Verification items for the finished model (mm, model axes). Face numbers are marked on the shaded views. Round coordinates to 2 decimals unless told otherwise and drop trailing zeros. Write each loop counter-clockwise with the first axis right and the second up, starting at its lowest first coordinate (ties: lowest second). Pieces come first, ordered by that corner, then holes. Notation, with made-up numbers: (62.25, -9.5) - (75.25, -9.5) arc R24 ccw to (75.25, 21.5) - close; hole circle Ø7 at (64, 19.5). An arc over 180 degrees is marked (long way). Answer as a JSON object with one key per item and string values. Group by question number.
1) Thickness scan on line 1 (X direction, y = -7, z = 2.2) (3 decimals); line 2 (X direction, y = 12.5, z = 2.4); line 3 (X direction, y = -5, z = 0.6). Record the ranges inside material, lowest first.
2) Mould release check, pull along Y, two halves, no side actions. Record for the marked faces 1, 2 and 3: +Y half, -Y half, draft (parallel to the pull), parting line (faces both ways), or undercut.
3) Section check A-A (y = 14). Enter the section's corners in (x, z), then the cut area to 3 significant figures.
4) Go/stop test with a flat-tipped pin: pin 1 Ø6 at (x, y) = (-12.12, -7) entering from +Z. Record where the tip stops, or that it passes through.
5) Section check D-D (x = 0). Enter the section's corners in (y, z), then the cut area to 4 significant figures.
6) Section check C-C (z = 1). Enter the section's corners in (x, y) (3 decimals), then the cut area to 3 significant figures.
7) Section check B-B (x = -11.5). Enter the section's corners in (y, z), then the cut area to 3 significant figures.
```python
from build123d import *

# Parameters (mm, degrees)
BOSS_EXTRU_2_DEPTH = 3


with BuildPart() as part:
    # Esquisse1 → Boss.-Extru.2 (new body)
    with BuildSketch(Plane.XY):
        with BuildLine():
            ThreePointArc((-12.288149304, -10.247018429), (0.000780623, -15.999999981), (12.289149128, -10.245819328))
            ThreePointArc((12.289149128, -10.245819328), (9.309773091, -5.375), (15.017714385, -5.519805672))
            ThreePointArc((15.017714385, -5.519805672), (13.856406461, 8), (2.728565257, 15.765625))
            ThreePointArc((2.728565257, 15.765625), (0, 10.75), (-2.728565257, 15.765625))
            ThreePointArc((-2.728565257, 15.765625), (-13.856384318, 8.000038352), (-15.01774494, -5.519722539))
            ThreePointArc((-15.01774494, -5.519722539), (-9.310492225, -5.375986513), (-12.288149304, -10.247018429))
        make_face()
    extrude(amount=BOSS_EXTRU_2_DEPTH)


solid = part.part
```
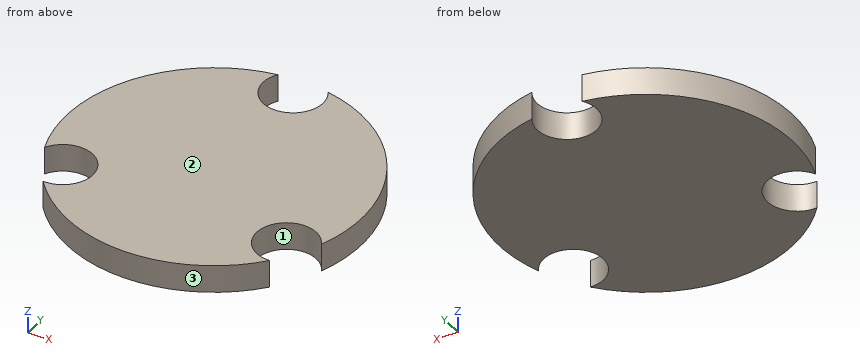
Returned:
{
 "1": {"line 1": "-8.875 to 8.874", "line 2": "-9.99 to -2.88, 2.88 to 9.99", "line 3": "-15.2 to -14.69, -9.56 to 9.56, 14.69 to 15.2"},
 "2": {"face 1": "undercut", "face 2": "draft", "face 3": "-Y half"},
 "3": {"outline": "(-7.75, 0) - (-3.25, 0) - (-3.25, 3) - (-7.75, 3) - close; (3.25, 0) - (7.75, 0) - (7.75, 3) - (3.25, 3) - close", "area": "27.0 mm2"},
 "4": {"pin 1": "through"},
 "5": {"outline": "(-16, 0) - (10.75, 0) - (10.75, 3) - (-16, 3) - close", "area": "80.25 mm2"},
 "6": {"outline": "(-15.018, -5.52) arc R3.25 cw (long way) to (-12.288, -10.247) arc R16 ccw to (12.289, -10.246) arc R3.25 cw (long way) to (15.018, -5.52) arc R16 ccw to (2.729, 15.766) arc R3.25 cw (long way) to (-2.729, 15.766) arc R16 ccw to start", "area": "719 mm2"},
 "7": {"outline": "(-11.12, 0) - (-10.19, 0) - (-10.19, 3) - (-11.12, 3) - close; (-3.81, 0) - (11.12, 0) - (11.12, 3) - (-3.81, 3) - close", "area": "47.6 mm2"}
}
